Job drawing, mm, ordinate dimensions from the low corner. One solid piece. Give positions to 0.01 mm unless a question says otherwise; leave off trailing zeros. Write each loop counter-clockwise with the first axis right and the second up, starting at its lowest first coordinate (ties: lowest second). Pieces come first, ordered by that corner, then holes. Notation, with made-up numbers: (-11.75, 73) - (3.25, 73) arc R7 ccw to (3.25, 77) - close; hole circle Ø4 at (2, 87.5). An arc over 180 degrees is marked (long way). Answer in a Markdown table with one row per item. Add a question column.
1. Probe line 1 along Y through (x, z) = (7.5, 10) (1 decimal); line 2 along Y through (x, z) = (14, 3.5) (1 decimal); line 3 along X through (y, z) = (17, 9.25) (1 decimal). List the from-to ranges inside material, lowest first.
2. Band-saw the part on C-C on z = 7.25. State how many separate pieces and enclosed holes the cut face has, plus the area to 3 significant figures.
3. Band-saw the part on B-B on y = 18.5. Write the cut outline in (x, z).
4. Band-saw the part on A-A on x = 17.8. Write the cut outline in (y, z).
5. Pull direction X, two halves, no side cores. Call the marked faces 1, 2 and 3: released by +X, released by -X, zero draft, split by the parting line, or undercut.
6. Drop flat-ended pins along their axis: pin 1 Ø5 at (x, y) = (13, 28.5) entering from -Z; pin 2 Ø3 at (x, y) = (21, 5) entering from -Z; pin 3 Ø5 at (y, z) = (6.5, 7.5) entering from +X; pin 4 Ø1.5 at (y, z) = (15, 2.5) entering from +X. Give the stop position or say it passes through.
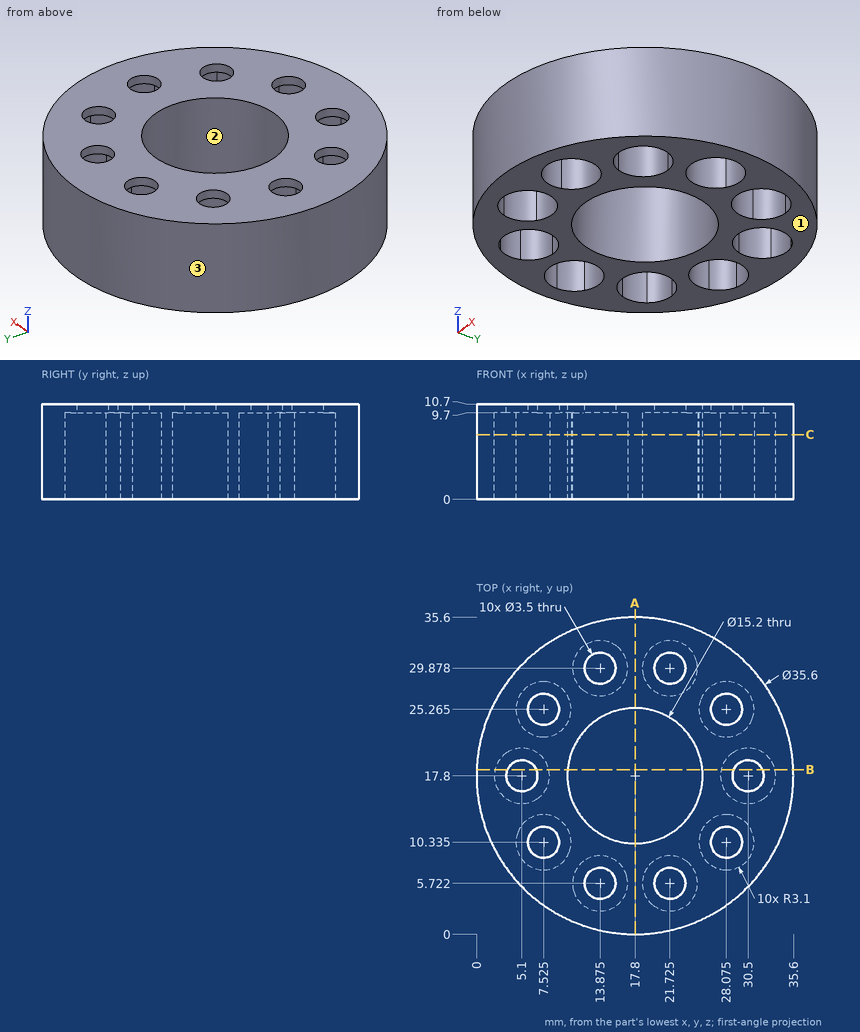
Values:
| question | item | result |
|---|---|---|
| 1 | line 1 | y = 3.3 to 8.6, 12.1 to 23.5, 27 to 32.3 |
| 1 | line 2 | y = 0.4 to 2.6, 8.8 to 11.2, 24.4 to 26.8, 33 to 35.2 |
| 1 | line 3 | x = 0 to 2.1, 8.1 to 10.2, 25.4 to 27.5, 33.5 to 35.6 |
| 2 | separate pieces | 1 |
| 2 | enclosed holes | 11 |
| 2 | area | 512 mm² |
| 3 | outline | (0.01, 0) - (2.08, 0) - (2.08, 9.7) - (3.5, 9.7) - (3.5, 10.7) - (0.01, 10.7) - close; (6.7, 9.7) - (8.12, 9.7) - (8.12, 0) - (10.23, 0) - (10.23, 10.7) - (6.7, 10.7) - close; (25.37, 0) - (27.48, 0) - (27.48, 9.7) - (28.9, 9.7) - (28.9, 10.7) - (25.37, 10.7) - close; (32.1, 9.7) - (33.52, 9.7) - (33.52, 0) - (35.59, 0) - (35.59, 10.7) - (32.1, 10.7) - close |
| 4 | outline | (0, 0) - (10.2, 0) - (10.2, 10.7) - (0, 10.7) - close; (25.4, 0) - (35.6, 0) - (35.6, 10.7) - (25.4, 10.7) - close |
| 5 | face 1 | zero draft |
| 5 | face 2 | undercut |
| 5 | face 3 | split by the parting line |
| 6 | pin 1 | stops at z = 0 |
| 6 | pin 2 | stops at z = 9.7 |
| 6 | pin 3 | stops at x = 33.27 |
| 6 | pin 4 | stops at x = 35.48 |
